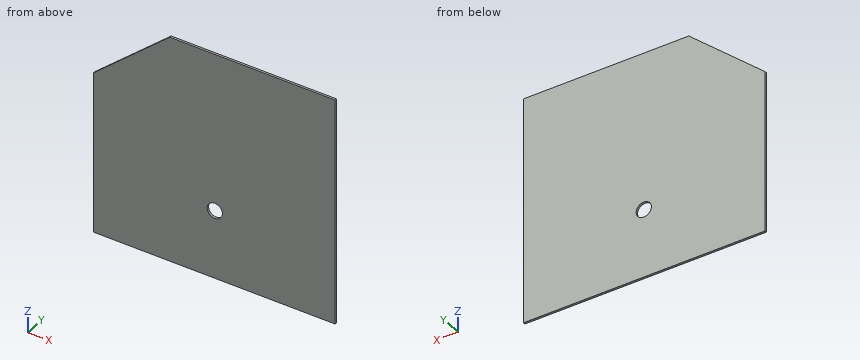
from build123d import *

# Parameters (mm, degrees)
SKETCH1_W           = 452.46
SKETCH1_H           = 425
BOSS_EXTRUDE1_DEPTH = 4
SKETCH2_R           = 14.275
CUT_EXTRUDE1_DEPTH  = 5
CUT_EXTRUDE2_DEPTH  = 5


with BuildPart() as part:
    # Sketch1 → Boss-Extrude1 (new body)
    with BuildSketch(Plane(origin=(0, 0, 0), x_dir=(1, 0, 0), z_dir=(0, 1, 0))):
        with Locations((12.58495796, 30.41049436)):
            Rectangle(SKETCH1_W, SKETCH1_H)
    extrude(amount=BOSS_EXTRUDE1_DEPTH)

    # Sketch2 → Cut-Extrude1 (cut, through all)
    with BuildSketch(Plane.XZ.offset(-4)):
        with Locations((13.51495796, -114.81049436)):
            Circle(SKETCH2_R)
    extrude(amount=CUT_EXTRUDE1_DEPTH, mode=Mode.SUBTRACT)

    # Sketch3 → Cut-Extrude2 (cut, through all)
    with BuildSketch(Plane(origin=(0, 4, 0), x_dir=(1, 0, 0), z_dir=(0, 1, 0))):
        Polygon((-70.791344552, -182.08950564), (-213.64504204, -59.421992734), (-317.358115476, -168.108607174), (-142.218193296, -320.092437945), align=None)
    extrude(amount=-CUT_EXTRUDE2_DEPTH, mode=Mode.SUBTRACT)


solid = part.part
Model file for the job. Use its own axes, mm. Give positions to 0.01 mm unless a question says otherwise; leave off trailing zeros. Order: outer loops, then holes, each group sorted by start corner. A loop starts at its lowest first (then second) coordinate and runs counter-clockwise, first axis right, second up. Notation, with made-up numbers: (52, -15) - (66, -15) arc R18 ccw to (66, -1) - close; hole circle Ø2 at (77, 60). An arc over 180 degrees is marked (long way). Return JSON: item names as keys, results as strings.
1) Cut at D-D, the plane x = -111.5. Give the cut face in (y, z).
Geometry says:
{"outline": "(0, -242.91) - (4, -242.91) - (4, 147.13) - (0, 147.13) - close"}
2) Cut at C-C, the plane x = -175.5. Give the cut face in (y, z).
Geometry says:
{"outline": "(0, -242.91) - (4, -242.91) - (4, 92.18) - (0, 92.18) - close"}
3) Probe line 1 (X direction, y = 3.35, z = 59.5); line 2 (Z direction, x = -161.5, y = 3.55); line 3 (X direction, y = 2.1, z = 144.5). List the from-to ranges inside material, lowest first. Write a range as from..to.
Geometry says:
{"line 1": "-213.55..238.81", "line 2": "-242.91..104.2", "line 3": "-114.57..238.81"}
4) Cut at A-A, the plane x = 6.5. Give the cut face in (y, z).
Geometry says:
{"outline": "(0, -242.91) - (4, -242.91) - (4, -127.24) - (0, -127.24) - close; (0, -102.38) - (4, -102.38) - (4, 182.09) - (0, 182.09) - close"}
